Model file for the job. Use its own axes, mm. Coordinates: 2 decimals unless noted, no trailing zeros. Order: outer loops, then holes, each group sorted by start corner. A loop starts at its lowest first (then second) coordinate and runs counter-clockwise, first axis right, second up. Notation, with made-up numbers: (87, 69.25) -> (105, 69.25) arc R26 cw to (105, 102.25) -> close; hole circle Ø11 at (50.25, 14). An arc over 180 degrees is marked (long way). Write item = value, one per line. Start each with the question number.
Q1. Cut at C-C, the plane z = 107. List the corners of the cut face in (x, y).
Q2. Flat gauge pins, fed straight in: pin 1 (2 mm diameter, centred on x = 21.5, z = 158.5, fed in from +Y); pin 2 (1.5 mm diameter, centred on x = 49.5, z = 97, fed in from +Y); pin 3 (10 mm diameter, centred on x = 40.5, z = 134, fed in from +Y); pin 4 (4 mm diameter, centred on x = -54.5, y = -58, fed in from +Z). Where does each tip first touch, or does it go through?
Q3. Wall check: line 1 (Z direction, x = 0, y = 15) (3 decimals); line 2 (X direction, y = -19, z = 173); line 3 (Y direction, x = -3.5, z = 75.5). Give the ranges that are in metal, low to high. Write a range as from..to.
Q4. Mould opens along Y. For faces 1 (the face through (1, 1, 0)), 2 (the face through (0, 0, 3.175)), 3 (the face through (-60.48, 19.05, 100)) say: +Y half, -Y half, draft (parallel to the pull), parting line (faces both ways), or undercut.
Q5. Cut at D-D, the plane z = 172.5. List the corners of the cut face in (x, y).
Q6. Cut at A-A, the plane y = 0. List the corners of the cut face in (x, z) (1 decimal), plus the area to 3 significant figures.
from build123d import *

# Parameters (mm, degrees)
F3_R = 1.5875


# Not quite as in the source:
# - a variable given as a bare number and used for a length is read in inches; the dataset says mm whatever the document's units were


with BuildPart() as f2:
    # F1 (on Front) → F2 (revolve)
    with BuildSketch(Plane.XZ):
        with BuildLine():
            Line((-50.8, 0), (0, 0))
            Line((0, 0), (0, 3.175))
            Line((0, 3.175), (-29.0172447749, 3.175))
            Line((-29.0172447749, 3.175), (-73.0551675175, 201.8488507874))
            ThreePointArc((-73.0551675175, 201.8488507874), (-74.8424777646, 203.1850293835), (-76.2, 201.4138759344))
            Line((-76.2, 201.4138759344), (-50.8, 0))
        make_face()
    revolve(axis=Axis((0, 0, 1.5875), (0, 0, -1)))

    # F3
    f3_edges = [f2.edges().sort_by_distance(p)[0] for p in [
        (50.8, 0, 0),
        (29.017245, 0, 3.175),
    ]]
    fillet(f3_edges, radius=F3_R)


solid = f2.part
Here are the results:
q1.outline = circle Ø128.59 at (0, 0); hole circle Ø104.06 at (0, 0)
q2.pin_1 = 67.78
q2.pin_2 = 39.97
q2.pin_3 = 57.73
q2.pin_4 = through
q3.line_1 = 0..3.175
q3.line_2 = -70.09..-63.9, 63.9..70.09
q3.line_3 = -60.22..-44.91, 44.91..60.22
q4.face_1 = draft
q4.face_2 = undercut
q4.face_3 = parting line
q5.outline = circle Ø145.11 at (0, 0); hole circle Ø133.1 at (0, 0)
q6.outline = (-76.2, 201.4) -> (-51, 1.4) arc R1.6 ccw to (-49.4, 0) -> (49.4, 0) arc R1.6 ccw to (51, 1.4) -> (76.2, 201.4) arc R1.6 ccw to (73.1, 201.8) -> (29.3, 4.4) arc R1.6 cw to (27.7, 3.2) -> (-27.7, 3.2) arc R1.6 cw to (-29.3, 4.4) -> (-73.1, 201.8) arc R1.6 ccw to start
q6.area = 5,370 mm²
